Can you work these out from the model? Positions are in its coordinate system, mm. A direction names the side the tool comes from. Coordinates: 2 decimals unless noted, no trailing zeros. Order: outer loops, then holes, each group sorted by start corner. A loop starts at its lowest first (then second) coordinate and runs counter-clockwise, first axis right, second up. Notation, with made-up numbers: (54, 22) -> (63, 22) arc R29 cw to (63, 55) -> close; hole circle Ø3 at (28, 14). An arc over 180 degrees is marked (long way). Answer in a Markdown table with one row per item. Add a question column.
1. Imagine slicing it at B-B on x = 42. Write out the boundary of the cut face in (y, z), plus the area to 3 significant figures.
2. If I drill on line 1 along Y through (x, z) = (12.5, 3); line 2 along X through (y, z) = (-9.5, 8); line 3 along X through (y, z) = (10, 0.75), over which ranges is the centre line in solid material (lowest first)? Write a range as [from, to].
3. Will these pins go through, and if not, where does the flat tip stop? pin 1 (3 mm diameter, centred on x = 39.5, z = 3, fed in from -Y); pin 2 (6 mm diameter, centred on y = -10, z = 4, fed in from -X); pin 3 (5 mm diameter, centred on y = -7.5, z = 4, fed in from +X).
4. On a 3-axis mill with a long thin cutter (end or side, diameter ignored), from which of +Z, -Z, +X, -X, +Y, -Y can I reach the whole of each face in a straight line? I mean faces 1 (the face through (-2.5, 7, 5)), 2 (the face through (1, 8, 0)), 3 (the face through (25, 21.976, 5)), 4 (the face through (-21, 0, 5)). Say none if no direction works.
5. Imagine slicing it at A-A on y = 12. Write out the boundary of the cut face in (x, z).
from build123d import *

# Parameters (mm, degrees)
F1_DEPTH = 10


with BuildPart() as f1:
    # F0 (on Top) → F1 (new body)
    with BuildSketch(Plane.XY):
        with BuildLine():
            Line((-2.5, -21.9755824495), (2.5, -21.9755824495))
            Line((2.5, -21.9755824495), (2.5, 21.9755824495))
            Line((2.5, 21.9755824495), (47.5, 21.9755824495))
            Line((47.5, 21.9755824495), (47.5, 26.9755824495))
            Line((47.5, 26.9755824495), (-2.5, 26.9755824495))
            Line((-2.5, 26.9755824495), (-2.5, 21.9755824495))
            Line((-2.5, 21.9755824495), (-2.5, -14.2228389159))
            add(Edge.make_bspline(
                [(-18.8081365824, 0), (-16.7830632678, -4.900555724), (-13.1043678113, -13.8027776567), (-5.7885545713, -14.0925723692), (-2.5, -14.2228389159)],
                knots=[0, 0, 0, 0, 0.5504868067, 1, 1, 1, 1], degree=3))
            Line((-18.8081365824, 0), (-23.8081365824, 0))
            add(Edge.make_bspline(
                [(-2.5, -21.9755824495), (-8.0809096282, -20.9474647123), (-17.3359240555, -16.3424369165), (-21.2225849489, -6.4176707959), (-23.8081365824, 0)],
                knots=[0, 0, 0, 0, 0.4808804759, 1, 1, 1, 1], degree=3))
        make_face()
    extrude(amount=F1_DEPTH)


solid = f1.part
Answers follow:
| question | item | result |
|---|---|---|
| 1 | outline | (21.98, 0) -> (26.98, 0) -> (26.98, 10) -> (21.98, 10) -> close |
| 1 | area | 50.0 mm² |
| 2 | line 1 | y = [21.98, 26.98] |
| 2 | line 2 | x = [-19.68, -14.1], [-2.5, 2.5] |
| 2 | line 3 | x = [-2.5, 2.5] |
| 3 | pin 1 | stops at y = 21.98 |
| 3 | pin 2 | stops at x = -20.89 |
| 3 | pin 3 | stops at x = 2.5 |
| 4 | face 1 | +Z, -Z, +Y |
| 4 | face 2 | -Z, +X, -X, +Y, -Y |
| 4 | face 3 | +Z, -Z, +X, -Y |
| 4 | face 4 | +Z, -Z, -X, +Y |
| 5 | outline | (-2.5, 0) -> (2.5, 0) -> (2.5, 10) -> (-2.5, 10) -> close |
